Part model, mm, in its own coordinate system. A direction names the side the tool comes from. Coordinates: 2 decimals unless noted, no trailing zeros. Loops run counter-clockwise (first coordinate to the right, second up) from the corner with the lowest first, then second, coordinate; pieces in that order, holes last. Notation, with made-up numbers: (70, 87) - (79, 87) arc R22 cw to (79, 115) - close; hole circle Ø10 at (9.5, 75). An arc over 180 degrees is marked (long way). Answer as CSV lines item,"result".
from build123d import *

# Parameters (mm, degrees)
F0_W     = 117.475
F0_H     = 117.475
F0_R     = 7.9375
F0_R_2   = 14.2875
F1_DEPTH = 6.35
F2_DEPTH = 38.1
F3_SIZE  = 0.5
F4_SIZE  = 0.5


with BuildPart() as f1:
    # F0 (on Top) → F1 (new body)
    with BuildSketch(Plane.XY):
        Rectangle(F0_W, F0_H)
        with Locations((-39.6875, -39.6875)):
            Circle(F0_R, mode=Mode.SUBTRACT)
        with Locations((39.6875, -39.6875)):
            Circle(F0_R, mode=Mode.SUBTRACT)
        Circle(F0_R_2, mode=Mode.SUBTRACT)
        with Locations((-39.6875, 39.6875)):
            Circle(F0_R, mode=Mode.SUBTRACT)
        with Locations((39.6875, 39.6875)):
            Circle(F0_R, mode=Mode.SUBTRACT)
        Polygon((63.2375, 58.7375), (58.7375, 58.7375), (58.7375, -58.7375), (-58.7375, -58.7375), (-58.7375, -63.2375), (63.2375, -63.2375), align=None)
        Polygon((71.4375, 58.7375), (63.2375, 58.7375), (63.2375, -63.2375), (-58.7375, -63.2375), (-58.7375, -71.4375), (71.4375, -71.4375), align=None)
    extrude(amount=F1_DEPTH)

    # F0 (on Top) → F2 (join)
    with BuildSketch(Plane.XY):
        Polygon((63.2375, 58.7375), (58.7375, 58.7375), (58.7375, -58.7375), (-58.7375, -58.7375), (-58.7375, -63.2375), (63.2375, -63.2375), align=None)
    extrude(amount=F2_DEPTH)

    # F3
    f3_edges = [f1.edges().sort_by_distance(p)[0] for p in [
        (31.75, -39.6875, 0),
        (-47.625, -39.6875, 0),
        (-47.625, 39.6875, 0),
        (31.75, 39.6875, 0),
        (-14.2875, 0, 0),
    ]]
    chamfer(f3_edges, length=F3_SIZE)

    # F4
    f4_edges = [f1.edges().sort_by_distance(p)[0] for p in [
        (-47.625, 39.6875, 6.35),
        (31.75, 39.6875, 6.35),
        (-14.2875, 0, 6.35),
        (31.75, -39.6875, 6.35),
        (-47.625, -39.6875, 6.35),
    ]]
    chamfer(f4_edges, length=F4_SIZE)


solid = f1.part
Q1. Saw through at B-B (x = 0). Give the cut face in (y, z), then the cut area to 3 significant figures.
Results:
outline,"(-71.44, 0) - (-14.79, 0) - (-14.29, 0.5) - (-14.29, 5.85) - (-14.79, 6.35) - (-58.74, 6.35) - (-58.74, 38.1) - (-63.24, 38.1) - (-63.24, 6.35) - (-71.44, 6.35) - close; (14.29, 0.5) - (14.79, 0) - (58.74, 0) - (58.74, 6.35) - (14.79, 6.35) - (14.29, 5.85) - close"
area,"788 mm^2"
Q2. Saw through at D-D (x = 16.5). Give the cut face in (y, z), then the cut area to 3 significant figures.
Results:
outline,"(-71.44, 0) - (58.74, 0) - (58.74, 6.35) - (-58.74, 6.35) - (-58.74, 38.1) - (-63.24, 38.1) - (-63.24, 6.35) - (-71.44, 6.35) - close"
area,"969 mm^2"
Q3. Saw through at A-A (y = 0). Give the cut face in (x, z).
Results:
outline,"(-58.74, 0) - (-14.79, 0) - (-14.29, 0.5) - (-14.29, 5.85) - (-14.79, 6.35) - (-58.74, 6.35) - close; (14.29, 0.5) - (14.79, 0) - (71.44, 0) - (71.44, 6.35) - (63.24, 6.35) - (63.24, 38.1) - (58.74, 38.1) - (58.74, 6.35) - (14.79, 6.35) - (14.29, 5.85) - close"
Q4. Which spindle directions (+Z, -Z, +X, -X, +Y, -Y) get a long thin tool onto all of the face, cutting with end or side? Do faces 1 (the face through (-58.738, -11, 6)), 2 (the face through (58.738, 1, 22)). Say none if no direction does.
Results:
face 1,"+Z, -Z, -X, +Y, -Y"
face 2,"+Z, -X, +Y"
Q5. Wall check: L1, parallel to X at y = 34.5, z = 6; L2, parallel to X at y = 1, z = 5.5; L3, parallel to X at y = -58, z = 16.5. Give the ranges that are in metal, low to high.
Results:
L1,"x = -58.74 to -45.89, -33.48 to 33.48, 45.89 to 71.44"
L2,"x = -58.74 to -14.25, 14.25 to 71.44"
L3,"x = 58.74 to 63.24"
Q6. Flat gauge pins, fed straight in: pin 1 (1.5 mm diameter, centred on x = 8.5, z = 11.5, fed in from +Y); pin 2 (1 mm diameter, centred on y = 16.5, z = 19, fed in from +X); pin 3 (8 mm diameter, centred on x = 25, z = 11, fed in from -Y). Where does each tip first touch, or does it go through?
Results:
pin 1,"stops at y = -58.74"
pin 2,"stops at x = 63.24"
pin 3,"stops at y = -63.24"
Q7. Two-plate mould, pull along Y, no slides. Class faces 3 (the face through (47.02, -42.73, 3.14)), 4 (the face through (1, -63.238, 22)), 5 (the face through (5, -20, 0)): released by +Y, released by -Y, zero draft, split by the parting line, or undercut.
Results:
face 3,"undercut"
face 4,"released by -Y"
face 5,"zero draft"
Q8. Saw through at C-C (y = -28). Give the cut face in (x, z), then the cut area to 3 significant figures.
Results:
outline,"(-58.74, 0) - (71.44, 0) - (71.44, 6.35) - (63.24, 6.35) - (63.24, 38.1) - (58.74, 38.1) - (58.74, 6.35) - (-58.74, 6.35) - close"
area,"969 mm^2"
